Source: CAD feature listing. Evaluate the final solid. Frame: model axes, mm. A direction names the side the tool comes from. Round coordinates to 2 decimals unless told otherwise and drop trailing zeros. Loops run counter-clockwise (first coordinate to the right, second up) from the corner with the lowest first, then second, coordinate; pieces in that order, holes last. Notation, with made-up numbers: M -35.75,-1 L 23.25,-1 A19 cw 23.25,30 Z; hole C -17,15.25 d8. An arc over 180 degrees is marked long. Answer as CSV lines item,"result". Start each with the question number.
```python
from build123d import *

# Parameters (mm, degrees)
SKETCH_1_R          = 10
EXTRUDE_1_DEPTH     = 3
SKETCH_2_R          = 4
CUT_EXTRUDE_1_DEPTH = 15.456832295
SKETCH_3_R          = 1.5
CUT_EXTRUDE_2_DEPTH = 15.456832295
EXTRUDE_START       = -3
EXTRUDE_3_DEPTH     = 3
CUT_EXTRUDE_3_DEPTH = 32.764760349
SKETCH_10_R         = 1.5
CUT_EXTRUDE_6_DEPTH = 32.764760349


with BuildPart() as part:
    # 草图1 → 凸台-拉伸1 (new body)
    with BuildSketch(Plane(origin=(0, 0, 0), x_dir=(1, 0, 0), z_dir=(0, 1, 0))):
        with Locations(Location((0, 0, 0), (0, 0, 270))):
            Circle(SKETCH_1_R)
    extrude(amount=EXTRUDE_1_DEPTH)

    # 草图2 → 切除-拉伸1 (cut, through all)
    with BuildSketch(Plane(origin=(0, 3, 0), x_dir=(1, 0, 0), z_dir=(0, 1, 0))):
        with Locations(Location((0, 0, 0), (0, 0, 270))):
            Circle(SKETCH_2_R)
    extrude(amount=-CUT_EXTRUDE_1_DEPTH, mode=Mode.SUBTRACT)

    # 草图3 → 切除-拉伸2 (cut, through all)
    with BuildSketch(Plane(origin=(0, 3, 0), x_dir=(1, 0, 0), z_dir=(0, 1, 0))):
        with Locations(Location((7, 0, 0), (0, 0, 270))):
            Circle(SKETCH_3_R)
        with Locations(Location((4.949747468, -4.949747468, 0), (0, 0, 270))):
            Circle(SKETCH_3_R)
        with Locations(Location((0, -7, 0), (0, 0, 270))):
            Circle(SKETCH_3_R)
        with Locations(Location((-4.949747468, -4.949747468, 0), (0, 0, 270))):
            Circle(SKETCH_3_R)
        with Locations(Location((-7, 0, 0), (0, 0, 270))):
            Circle(SKETCH_3_R)
        with Locations(Location((0, 7, 0), (0, 0, 270))):
            Circle(SKETCH_3_R)
    extrude(amount=-CUT_EXTRUDE_2_DEPTH, mode=Mode.SUBTRACT)

    # 草图6 → 凸台-拉伸3 (add)
    with BuildSketch(Plane(origin=(0, 3, 0), x_dir=(1, 0, 0), z_dir=(0, 1, 0)).offset(EXTRUDE_START)):
        with BuildLine():
            Line((0, 10), (-30, 10))
            Line((-30, 10), (-30, -10))
            Line((-30, -10), (0, -10))
            ThreePointArc((0, -10), (-10, 0), (0, 10))
        make_face()
    extrude(amount=EXTRUDE_3_DEPTH)

    # 草图7 → 切除-拉伸3 (cut, through all)
    with BuildSketch(Plane(origin=(0, 3, 0), x_dir=(1, 0, 0), z_dir=(0, 1, 0))):
        Polygon((-30, 4.125285706), (-12.506803088, 7.04081822), (-13, 10), (-30, 10), align=None)
    extrude(amount=-CUT_EXTRUDE_3_DEPTH, mode=Mode.SUBTRACT)

    # 草图10 → 切除-拉伸6 (cut, through all)
    with BuildSketch(Plane.XZ):
        with Locations(Location((-25.658723667, 5.289102386, 0), (0, 0, 270))):
            Circle(SKETCH_10_R)
    extrude(amount=-CUT_EXTRUDE_6_DEPTH, mode=Mode.SUBTRACT)


solid = part.part
```
1) Ray query, line 1 along X through (y, z) = (1.7, 0); line 2 along X through (y, z) = (1.15, 6); line 3 along Z through (x, y) = (-25.5, 2). Return the intervals inside material, ascending.
2) Section A-A, the plane z = 0. Return loops of the section in (x, y).
3) Section B-B, the plane x = 4.5. Return loops of the section in (y, z), and give its area (3 significant figures).
4) Contact query for flat-ended pins moving along their axis: pin 1 Ø2.5 at (x, z) = (-4.95, 4.95) entering from -Y; pin 2 Ø1 at (y, z) = (1, 5) entering from +X. Output: stop coordinate, or through.
5) Access query for faces 4 (the cylindrical face through (10, 1, 0)), 5 (the flat face through (-12.75, 1.52, -8.5)). Directions: +Z, -Z, +X, -X, +Y, -Y. A direction counts if a zero-diameter tool reaches every point of the face in a straight line with its end or side. Return the directions, or none.
6) Section D-D, the plane z = -8. Return loops of the section in (x, y), and give its area (3 significant figures).
7) Section C-C, the plane y = 2.2. Give the number of separate pieces and of enclosed holes in the cut face, and give its area (3 significant figures).
8) Mould query, pull axis Z, two halves, no side actions, for faces 1 (the cylindrical face through (-24.17, 1.48, 5.48)), 2 (the flat face through (-6, 1, -10)), 3 (the flat face through (-30, 1, 3)). Classes: pulls with the +Z half, pulls with the -Z half, needs draft (parallel to the pull), parting line crosses it, or undercut.
Findings below:
1,line 1,"-30 to -8.5, -5.5 to -4, 4 to 5.5, 8.5 to 10"
1,line 2,"-30 to -26.98, -24.34 to -6.02, -3.88 to -1.12, 1.12 to 3.88, 6.02 to 8"
1,line 3,"-4.88 to 3.8, 6.78 to 10"
2,outline,"M -30,0 L -8.5,0 L -8.5,3 L -30,3 Z; M -5.5,0 L -4,0 L -4,3 L -5.5,3 Z; M 4,0 L 5.5,0 L 5.5,3 L 4,3 Z; M 8.5,0 L 10,0 L 10,3 L 8.5,3 Z"
3,outline,"M 0,-8.93 L 3,-8.93 L 3,3.52 L 0,3.52 Z; M 0,6.38 L 3,6.38 L 3,8.93 L 0,8.93 Z"
3,area,"45.0 mm²"
4,pin 1,"through"
4,pin 2,"x = 8.93"
5,face 4,"+X, +Y, -Y"
5,face 5,"-X, +Y, -Y"
6,outline,"M -12.67,0 L -1.12,0 L -1.12,3 L -12.67,3 Z; M 1.12,0 L 6,0 L 6,3 L 1.12,3 Z"
6,area,"49.3 mm²"
7,separate pieces,"1"
7,enclosed holes,"8"
7,area,"581 mm²"
8,face 1,"undercut"
8,face 2,"pulls with the -Z half"
8,face 3,"needs draft"
